Input: part model. Units: mm. Frame: model coordinates. Coordinates: 2 decimals unless noted, no trailing zeros. Loops run counter-clockwise (first coordinate to the right, second up) from the corner with the lowest first, then second, coordinate; pieces in that order, holes last. Notation, with made-up numbers: (16.5, 74) - (66.5, 74) arc R21 cw to (66.5, 105) - close; hole circle Ø6 at (-31.5, 28.5). An arc over 180 degrees is marked (long way). Use a Markdown table: item, result. Add a question column.
1. Draft query along Y for faces 1 (the face through (0.209, -9.523, 1.252)), 2 (the face through (-22.025, -99.184, 1.252)), 3 (the face through (-1, 24, 2.54)). Return one class per face: released by +Y, released by -Y, zero draft, split by the parting line, or undercut.
2. Section query D-D on y = 32. Return the cut outline in (x, z) (3 decimals), then the cut area to 3 significant figures.
3. Section query C-C on y = -40. Return the cut outline in (x, z), then the cut area to 3 significant figures.
4. Ray query, L1, parallel to Y at x = 1, z = 2.3; L2, parallel to X at y = 54, z = 0.55 (3 decimals); L3, parallel to X at y = -8, z = 1.7. Return the intervals inside material, ascending. Write a range as [from, to].
5. Contact query for flat-ended pins moving along their axis: P1, Ø1.5, axis at y = -42.5, z = 1.5, coming from the +X side; P2, Ø0.8, axis at y = 38, z = 1, coming from the -X side; P3, Ø1.5, axis at x = 74.5, z = 0.5, coming from the +Y side. Output: stop coordinate, or through.
6. Section query B-B on z = 1. Return the cut outline in (x, y) (3 decimals).
7. Section query A-A on x = 0. Return the cut outline in (y, z) (3 decimals).
```python
from build123d import *

# Parameters (mm, degrees)
SKETCH1_R           = 101.6
SKETCH1_R_2         = 4.24957387
BOSS_EXTRUDE1_DEPTH = 2.54


with BuildPart() as part:
    # Sketch1 → Boss-Extrude1 (new body)
    with BuildSketch(Plane.XY):
        Circle(SKETCH1_R)
        Circle(SKETCH1_R_2, mode=Mode.SUBTRACT)
        with BuildLine():
            Line((-9.525, 0), (-9.525, 75.602343714))
            ThreePointArc((-9.525, 75.602343714), (0, -76.2), (9.525, 75.602343714))
            Line((9.525, 75.602343714), (9.525, 0))
            ThreePointArc((9.525, 0), (0, -9.525), (-9.525, 0))
        make_face(mode=Mode.SUBTRACT)
    extrude(amount=BOSS_EXTRUDE1_DEPTH)


solid = part.part
```
Resolved:
| question | item | result |
|---|---|---|
| 1 | face 1 | undercut |
| 1 | face 2 | split by the parting line |
| 1 | face 3 | zero draft |
| 2 | outline | (-96.429, 0) - (-69.155, 0) - (-69.155, 2.54) - (-96.429, 2.54) - close; (-9.525, 0) - (9.525, 0) - (9.525, 2.54) - (-9.525, 2.54) - close; (69.155, 0) - (96.429, 0) - (96.429, 2.54) - (69.155, 2.54) - close |
| 2 | area | 187 mm² |
| 3 | outline | (-93.39, 0) - (-64.86, 0) - (-64.86, 2.54) - (-93.39, 2.54) - close; (64.86, 0) - (93.39, 0) - (93.39, 2.54) - (64.86, 2.54) - close |
| 3 | area | 145 mm² |
| 4 | L1 | [-101.6, -76.19], [-9.47, -4.13], [4.13, 101.6] |
| 4 | L2 | [-86.061, -53.763], [-9.525, 9.525], [53.763, 86.061] |
| 4 | L3 | [-101.28, -75.78], [-5.17, 5.17], [75.78, 101.28] |
| 5 | P1 | x = 92.63 |
| 5 | P2 | x = -94.39 |
| 5 | P3 | y = 69.88 |
| 6 | outline | circle Ø203.2 at (0, 0); hole (-9.525, 0) - (-9.525, 75.602) arc R76.2 ccw (long way) to (9.525, 75.602) - (9.525, 0) arc R9.525 cw to start; hole circle Ø8.499 at (0, 0) |
| 7 | outline | (-101.6, 0) - (-76.2, 0) - (-76.2, 2.54) - (-101.6, 2.54) - close; (-9.525, 0) - (-4.25, 0) - (-4.25, 2.54) - (-9.525, 2.54) - close; (4.25, 0) - (101.6, 0) - (101.6, 2.54) - (4.25, 2.54) - close |
